Input: part model. Units: mm. Frame: model coordinates. A direction names the side the tool comes from. Coordinates: 2 decimals unless noted, no trailing zeros. Loops run counter-clockwise (first coordinate to the right, second up) from the corner with the lowest first, then second, coordinate; pieces in that order, holes last. Notation, with made-up numbers: (-34, 12) - (13, 12) arc R18 ccw to (13, 45) - close; hole circle Ø2 at (-38.75, 75.5). An arc over 180 degrees is marked (long way). Use one line per item in the form item = value.
from build123d import *

# Parameters (mm, degrees)
SKETCH1_R           = 34.5
BOSS_EXTRUDE1_DEPTH = 3
SKETCH3_W           = 13.9
SKETCH3_H           = 13.9
CUT_EXTRUDE1_DEPTH  = 49.88251221
SKETCH4_R           = 12.627177327
CUT_EXTRUDE2_DEPTH  = 49.88251221
SKETCH5_W           = 5
SKETCH5_H           = 5
CUT_EXTRUDE3_DEPTH  = 1.5


with BuildPart() as part:
    # Sketch1 → Boss-Extrude1 (new body)
    with BuildSketch(Plane(origin=(0, 0, 0), x_dir=(1, 0, 0), z_dir=(0, 1, 0))):
        with Locations(Location((0, 0, 0), (0, 0, 270))):
            Circle(SKETCH1_R)
    extrude(amount=BOSS_EXTRUDE1_DEPTH)

    # Sketch3 → Cut-Extrude1 (cut, through all)
    with BuildSketch(Plane(origin=(0, 3, 0), x_dir=(1, 0, 0), z_dir=(0, 1, 0))):
        with Locations((23.105624339, -0.103761809)):
            Rectangle(SKETCH3_W, SKETCH3_H)
        with Locations((0.103761809, 23.105624339)):
            Rectangle(SKETCH3_W, SKETCH3_H)
        with Locations((-0.103761809, -23.105624339)):
            Rectangle(SKETCH3_W, SKETCH3_H)
        with Locations((-23.105624339, 0.103761809)):
            Rectangle(SKETCH3_W, SKETCH3_H)
    extrude(amount=-CUT_EXTRUDE1_DEPTH, mode=Mode.SUBTRACT)

    # Sketch4 → Cut-Extrude2 (cut, through all)
    with BuildSketch(Plane(origin=(0, 3, 0), x_dir=(1, 0, 0), z_dir=(0, 1, 0))):
        with Locations(Location((0, 0, 0), (0, 0, 270))):
            Circle(SKETCH4_R)
    extrude(amount=-CUT_EXTRUDE2_DEPTH, mode=Mode.SUBTRACT)

    # Sketch5 → Cut-Extrude3 (cut)
    with BuildSketch(Plane(origin=(0, 3, 0), x_dir=(1, 0, 0), z_dir=(0, 1, 0))):
        with Locations((19.603168608, 19.636741271)):
            Rectangle(SKETCH5_W, SKETCH5_H)
        with Locations((-19.636741271, 19.603168608)):
            Rectangle(SKETCH5_W, SKETCH5_H)
        with Locations((19.636741271, -19.603168608)):
            Rectangle(SKETCH5_W, SKETCH5_H)
        with Locations((-19.603168608, -19.636741271)):
            Rectangle(SKETCH5_W, SKETCH5_H)
    extrude(amount=-CUT_EXTRUDE3_DEPTH, mode=Mode.SUBTRACT)


solid = part.part
Q1. Cut plane A-A, the plane z = 0. Return loops of the section in (x, y).
Check values:
outline = (-34.5, 0) - (-30.06, 0) - (-30.06, 3) - (-34.5, 3) - close; (-16.16, 0) - (-12.63, 0) - (-12.63, 3) - (-16.16, 3) - close; (12.63, 0) - (16.16, 0) - (16.16, 3) - (12.63, 3) - close; (30.06, 0) - (34.5, 0) - (34.5, 3) - (30.06, 3) - close
Q2. Cut plane D-D, the plane x = 0. Return loops of the section in (y, z), then the cut area to 3 significant figures.
Check values:
outline = (0, -34.5) - (3, -34.5) - (3, -30.06) - (0, -30.06) - close; (0, -16.16) - (3, -16.16) - (3, -12.63) - (0, -12.63) - close; (0, 12.63) - (3, 12.63) - (3, 16.16) - (0, 16.16) - close; (0, 30.06) - (3, 30.06) - (3, 34.5) - (0, 34.5) - close
area = 47.8 mm²
Q3. Set-up query: faces 3 (the flat face through (-30.056, 2, 0)), 4 (the flat face through (-22.103, 2, 20)). Return all of +Z, -Z, +X, -X, +Y, -Y with unobstructed straight access to the full face (end or side cutting, diameter ignored); none if empty.
Check values:
face_3 = +Y, -Y
face_4 = +Y
Q4. Cut plane C-C, the plane y = 0.45. Return loops of the section in (x, z), then the cut area to 3 significant figures.
Check values:
outline = circle Ø69 at (0, 0); hole (-30.06, -7.05) - (-16.16, -7.05) - (-16.16, 6.85) - (-30.06, 6.85) - close; hole circle Ø25.25 at (0, 0); hole (-7.05, 16.16) - (6.85, 16.16) - (6.85, 30.06) - (-7.05, 30.06) - close; hole (-6.85, -30.06) - (7.05, -30.06) - (7.05, -16.16) - (-6.85, -16.16) - close; hole (16.16, -6.85) - (30.06, -6.85) - (30.06, 7.05) - (16.16, 7.05) - close
area = 2,470 mm²
Q5. First-contact query: P1, Ø0.9, axis at x = 1, y = 1.5, coming from the +Z side; P2, Ø1.6, axis at y = 2.5, z = -18.5, coming from the +X side; P3, Ø0.9, axis at x = -24.5, y = 2, coming from the +Z side; P4, Ø0.9, axis at x = -0.5, y = 2, coming from the -Z side. Flat tips, straight axial feed; report the tip coordinate or a pass-through.
Check values:
P1 = 34.5
P2 = 29.61
P3 = 24.74
P4 = -34.5
Q6. Ray query, line 1 along X through (y, z) = (0.9, 0); line 2 along X through (y, z) = (1.5, 26.5); line 3 along X through (y, z) = (0.45, -1.5). Return the intervals inside material, ascending. Write a range as [from, to].
Check values:
line_1 = [-34.5, -30.06], [-16.16, -12.63], [12.63, 16.16], [30.06, 34.5]
line_2 = [-22.09, -7.05], [6.85, 22.09]
line_3 = [-34.47, -30.06], [-16.16, -12.54], [12.54, 16.16], [30.06, 34.47]
Q7. Cut plane B-B, the plane x = 20. Return loops of the section in (y, z).
Check values:
outline = (0, -28.11) - (3, -28.11) - (3, -22.14) - (1.5, -22.14) - (1.5, -17.14) - (3, -17.14) - (3, -6.85) - (0, -6.85) - close; (0, 7.05) - (3, 7.05) - (3, 17.1) - (1.5, 17.1) - (1.5, 22.1) - (3, 22.1) - (3, 28.11) - (0, 28.11) - close
Q8. Pull-direction query (X, two-part tool) for faces 1 (the flat face through (0, 2, 30.056)), 2 (the cylindrical face through (1.517, 1.479, -34.467)); classes: pulls with the +X half, pulls with the -X half, needs draft (parallel to the pull), parting line crosses it, or undercut.
Check values:
face_1 = undercut
face_2 = parting line crosses it
